```python
from build123d import *

# Parameters (mm, degrees)
SKETCH1_R           = 3
SKETCH1_R_2         = 1.5
BOSS_EXTRUDE1_DEPTH = 5
FILLET1_R           = 2


with BuildPart() as part:
    # Sketch1 → Boss-Extrude1 (new body)
    with BuildSketch(Plane.XY):
        Polygon((-20, 45), (20, 45), (59.431325943, 63.387129258), (40, 10), (40, -10), (59.431325943, -63.387129258), (20, -45), (-20, -45), (-59.431325943, -63.387129258), (-40, -10), (-40, 10), (-59.431325943, 63.387129258), align=None)
        with Locations((-22.5, 30)):
            Circle(SKETCH1_R, mode=Mode.SUBTRACT)
        Circle(SKETCH1_R_2, mode=Mode.SUBTRACT)
        with Locations((-18, 0)):
            Circle(SKETCH1_R_2, mode=Mode.SUBTRACT)
        with Locations((18, 0)):
            Circle(SKETCH1_R_2, mode=Mode.SUBTRACT)
        with Locations((22.5, 30)):
            Circle(SKETCH1_R, mode=Mode.SUBTRACT)
        with Locations((22.5, -30)):
            Circle(SKETCH1_R, mode=Mode.SUBTRACT)
        with Locations((-22.5, -30)):
            Circle(SKETCH1_R, mode=Mode.SUBTRACT)
    extrude(amount=BOSS_EXTRUDE1_DEPTH)

    # Fillet1
    fillet1_edges = [part.edges().sort_by_distance(p)[0] for p in [
        (59.431325943, 63.387129258, 2.5),
        (59.431325943, -63.387129258, 2.5),
        (-59.431325943, -63.387129258, 2.5),
        (-59.431325943, 63.387129258, 2.5),
    ]]
    fillet(fillet1_edges, radius=FILLET1_R)


solid = part.part
```
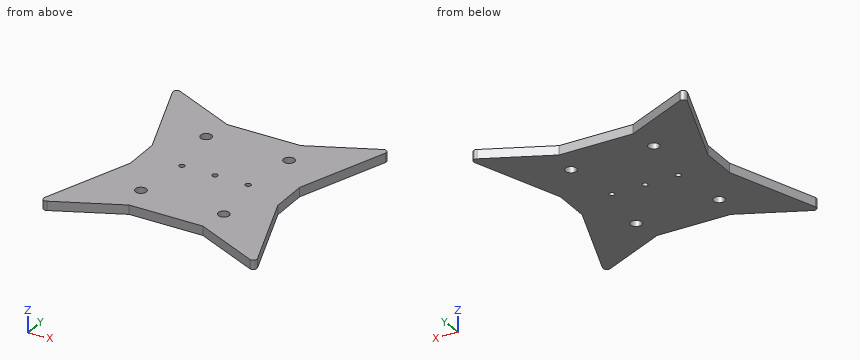
Build history of the part. All positions in model axes, mm. Coordinates: 2 decimals unless noted, no trailing zeros. Write each loop counter-clockwise with the first axis right and the second up, starting at its lowest first coordinate (ties: lowest second). Pieces come first, ordered by that corner, then holes.
1. Drill centre lines: probe 1 along Y at (x, z) = (-18, 2.95); probe 2 along Y at (x, z) = (22, 0.8); probe 3 along X at (y, z) = (32.5, 0.5). Where is each one in solid material? Low to high.
Answer block:
probe 1: y = -45 to -1.5, 1.5 to 45
probe 2: y = -45.93 to -32.96, -27.04 to 27.04, 32.96 to 45.93
probe 3: x = -48.19 to -24.16, -20.84 to 20.84, 24.16 to 48.19
2. Band-saw the part on B-B, the plane z = 3.2. Give the cut face in (x, y).
Answer block:
outline: (-57.78, -58.85) arc R2 ccw to (-55.06, -61.35) - (-20, -45) - (20, -45) - (55.06, -61.35) arc R2 ccw to (57.78, -58.85) - (40, -10) - (40, 10) - (57.78, 58.85) arc R2 ccw to (55.06, 61.35) - (20, 45) - (-20, 45) - (-55.06, 61.35) arc R2 ccw to (-57.78, 58.85) - (-40, 10) - (-40, -10) - close; hole circle Ø6 at (-22.5, -30); hole circle Ø6 at (-22.5, 30); hole circle Ø3 at (-18, 0); hole circle Ø3 at (0, 0); hole circle Ø3 at (18, 0); hole circle Ø6 at (22.5, -30); hole circle Ø6 at (22.5, 30)
3. Band-saw the part on C-C, the plane y = 30. Give the cut face in (x, z), and give its area (3 significant figures).
Answer block:
outline: (-47.28, 0) - (-25.5, 0) - (-25.5, 5) - (-47.28, 5) - close; (-19.5, 0) - (19.5, 0) - (19.5, 5) - (-19.5, 5) - close; (25.5, 0) - (47.28, 0) - (47.28, 5) - (25.5, 5) - close
area: 413 mm2
4. Band-saw the part on A-A, the plane x = 0. Give the cut face in (y, z).
Answer block:
outline: (-45, 0) - (-1.5, 0) - (-1.5, 5) - (-45, 5) - close; (1.5, 0) - (45, 0) - (45, 5) - (1.5, 5) - close
5. Drop flat-ended pins along their axis: pin 1 (2 mm diameter, centred on y = 41, z = 2, fed in from +X); pin 2 (5.5 mm diameter, centred on x = -22.5, y = -30, fed in from +Z); pin 3 (2 mm diameter, centred on y = 16, z = 1, fed in from -X); pin 4 (1.5 mm diameter, centred on y = 4.5, z = 2, fed in from -X). Give the stop position or say it passes through.
Answer block:
pin 1: stops at x = 51.65
pin 2: passes through
pin 3: stops at x = -42.55
pin 4: stops at x = -40
6. Band-saw the part on D-D, the plane y = 49. Give the cut face in (x, z).
Answer block:
outline: (-54.19, 0) - (-28.58, 0) - (-28.58, 5) - (-54.19, 5) - close; (28.58, 0) - (54.19, 0) - (54.19, 5) - (28.58, 5) - close
